Autodesk Inventor part; units mm, degrees
ref_plane "YZ Plane" through (0, 0, 0) normal (1, 0, 0) x (0, 1, 0)
ref_plane "XZ Plane" through (0, 0, 0) normal (0, 1, 0) x (-1, 0, 0)
ref_plane "XY Plane" through (0, 0, 0) normal (0, 0, 1) x (1, 0, 0)
sketch "Sketch1" plane through (0, 0, 0) normal (0, 0, 1) x (1, 0, 0)
  line L0 (-7.898, 5.9756) -> (42.102, 5.9756)
  line L1 (42.102, 5.9756) -> (42.102, -14.0244)
  line L2 (42.102, -14.0244) -> (-7.898, -14.0244)
  line L3 (-7.898, -14.0244) -> (-7.898, 5.9756)
  point P0 (0, 0)
  dimension "d0" = 50
  dimension "d1" = 20
extrude "Extrusion1" add sketch "Sketch1" along normal blind 10
sketch "Sketch2" plane through (0, 0, 10) normal (0, 0, 1) x (1, 0, 0)
  line L0 (-7.898, 5.9756) -> (-7.898, -14.0244)
  line L1 (-7.898, 4.3731) -> (42.102, -9.0244)
  line L2 (42.102, -14.0244) -> (42.102, 5.9756)
  line L3 (-7.898, 4.3731) -> (-7.898, 5.9756)
  line L4 (42.102, 5.9756) -> (-7.898, 5.9756)
  line L5 (42.102, 5.9756) -> (42.102, -9.0244)
  point P0 (0, 0)
  dimension "d4" = 5
  dimension "d5" = 75
extrude "Extrusion2" cut sketch "Sketch2" against normal up to surface (10 mm away)
sketch "Sketch3" plane through (-7.898, 4.3731, 10) normal (0.258819, 0.9659258, 0) x (0.9659258, -0.258819, 0)
  line L0 (53.0579, 0) -> (51.7638, 0)
  line L1 (0, 10) -> (4.7616, 10)
  line L2 (51.7638, 0) -> (0, 0)
  line L3 (0, 0) -> (0, 10)
  line L4 (0, 10) -> (51.7638, 10)
  line L5 (51.7638, 10) -> (51.7638, 0)
  point P0 (8.7608, 10)
extrude "Extrusion3" add sketch "Sketch3" along normal blind 10
sketch "Sketch4" plane through (-5.3099, 14.0324, 10) normal (0.258819, 0.9659258, 0) x (0.9659258, -0.258819, 0)
  line L0 (48.632, 0) -> (3.132, 0)
  line L1 (3.132, 0) -> (3.132, 6)
  line L2 (3.132, 6) -> (48.632, 6)
  line L3 (48.632, 6) -> (48.632, 0)
  line L4 (0, 0) -> (51.7638, 0)
  line L5 (0, 10) -> (0, 0)
  line L6 (51.7638, 10) -> (0, 10)
  point P0 (8.7608, 10)
  point P1 (25.882, 5)
  dimension "d10" = 45.5
  dimension "d11" = 6
  dimension "d13" = 25.882
  dimension "d14" = 22.75
  dimension "d23" = 0
extrude "Extrusion4" cut sketch "Sketch4" against normal blind 5.5
sketch "Sketch5" plane through (0, 0, 10) normal (0, 0, 1) x (1, 0, 0)
  line L0 (0, -5.2088) -> (0, -10.2088)
  line L1 (0, -10.2088) -> (-4.3301, -7.7088)
  line L2 (-4.3301, -7.7088) -> (0, -5.2088)
  point P0 (0, 0)
  dimension "d17" = 5
  dimension "d18" = 5
extrude "Extrusion5" cut sketch "Sketch5" against normal blind 2.5
properties part number "Angled Base AdapterFront"
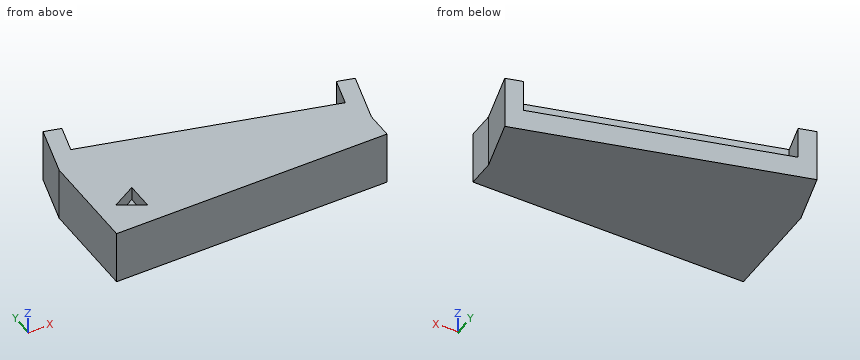
Verification items for the finished model (mm, model axes). Give positions to 0.01 mm unless a question says otherwise; leave off trailing zeros. Order: outer loops, then holes, each group sorted by start corner. A loop starts at its lowest first (then second) coordinate and runs counter-clockwise, first axis right, second up. Notation, with made-up numbers: M 7.5,49.25 L 34.5,49.25 A14 cw 34.5,74.25 Z; hole C 61,-34 d11. An arc over 180 degrees is marked long. Use one line per item in the form item = value. Start each with the question number.
Q1. Section check C-C (z = 4.5). Enter the section's corners in (x, y) (1 decimal).
Q2. Section check A-A (z = 8.5). Enter the section's corners in (x, y) (1 decimal), then the cut area to 3 significant figures.
Q3. Scan lines: line 1 along X through (y, z) = (-11.75, 6); line 2 along Z through (x, y) = (8, 5.5); line 3 along Y through (x, z) = (23.5, 3.25). Record each from-to range of solid material in increasing order. Write a range as [from, to].
Q4. Section check D-D (x = 20). Enter the section's corners in (y, z), then the cut area to 3 significant figures.
Q5. Section check B-B (y = -11.75). Enter the section's corners in (x, z).
Q6. Go/stop test with flat-tipped pins: pin 1 Ø2.5 at (y, z) = (-11, 7.5) entering from +X; pin 2 Ø13.5 at (x, y) = (10, 5.5) entering from +Z; pin 3 Ø5 at (x, z) = (10.5, 3.5) entering from +Y. Record where each tip stops, or that it passes through.
Evaluation:
q1.outline = M -7.9,-14 L 42.1,-14 L 42.1,-9 L 44.7,0.6 L 41.7,1.4 L 40.2,-3.9 L -3.7,7.9 L -2.3,13.2 L -5.3,14 L -7.9,4.4 Z
q2.outline = M -7.9,-14 L 42.1,-14 L 42.1,-9 L 44.7,0.6 L 41.7,1.4 L 40.2,-3.9 L -3.7,7.9 L -2.3,13.2 L -5.3,14 L -7.9,4.4 Z; hole M -4.3,-7.7 L 0,-10.2 L 0,-5.2 Z
q2.area = 841 mm2
q3.line_1 = [-7.9, 42.1]
q3.line_2 = [0, 4]
q3.line_3 = [-14.02, 6.31]
q4.outline = M -14.02,0 L 7.25,0 L 7.25,4 L 1.55,4 L 1.55,10 L -14.02,10 Z
q4.area = 179 mm2
q5.outline = M -7.9,0 L 42.1,0 L 42.1,10 L -7.9,10 Z
q6.pin_1 = 42.1
q6.pin_2 = 10
q6.pin_3 = 10.47
